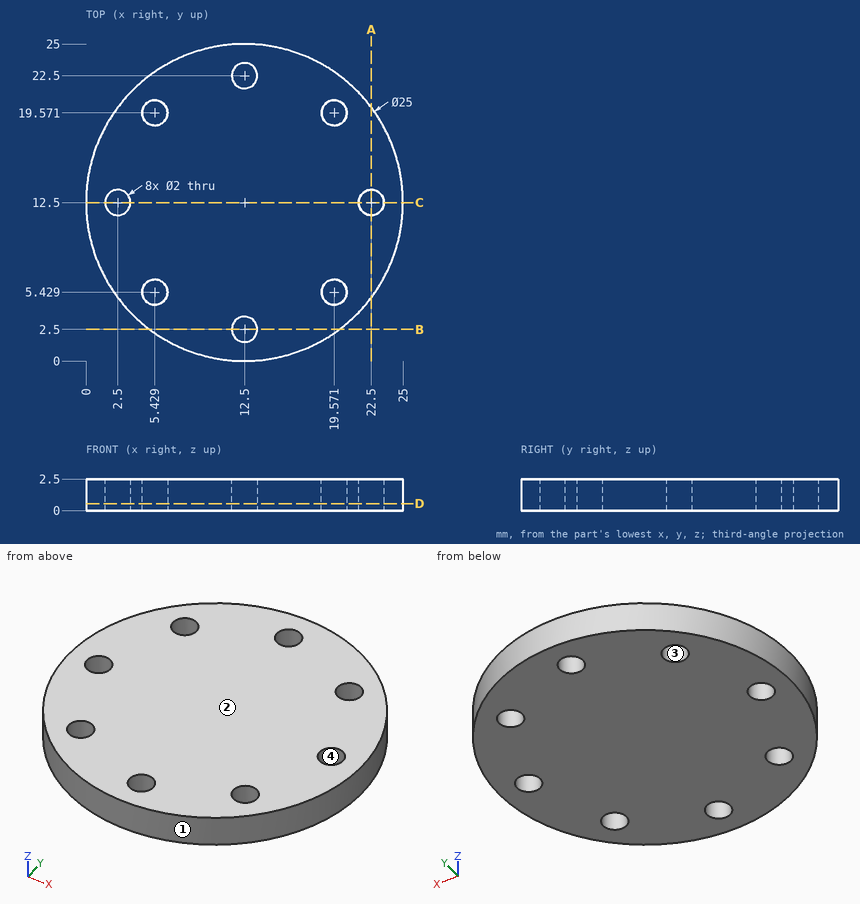
Geometry check sheet. Reference: drawing and pictorial views, mm from the part's lowest x, y, z. Give positions to 0.01 mm unless a question says otherwise; leave off trailing zeros. Order: outer loops, then holes, each group sorted by start corner. A loop starts at its lowest first (then second) coordinate and runs counter-clockwise, first axis right, second up.
1. Section check D-D, the plane z = 0.55. Give the number of separate pieces and of enclosed holes in the cut face, and give its area (3 significant figures).
2. Release check for a two-part mould opening along X. For the marked faces 1, 2, 3 and 4 record: pulls with the +X half, pulls with the -X half, needs draft (parallel to the pull), parting line crosses it, or undercut.
3. Thickness scan on L1, parallel to Y at x = 12.5, z = 0.25; L2, parallel to Y at x = 11.75, z = 0.2; L3, parallel to X at y = 18.75, z = 1.65 (1 decimal). Record the ranges inside material, lowest first.
4. Section check A-A, the plane x = 22.5. Enter the section's corners in (y, z), and give its area (3 significant figures).
5. Gauge pin test, flat end, axial feed: pin 1 Ø1 at (y, z) = (9.5, 1.5) entering from +X. Record the tip position at first contact, or that the pin passes through.
6. Section check C-C, the plane y = 12.5. Enter the section's corners in (x, z).
Values follow:
1. separate pieces: 1
1. enclosed holes: 8
1. area: 466 mm2
2. face 1: parting line crosses it
2. face 2: needs draft
2. face 3: undercut
2. face 4: undercut
3. L1: y = 0 to 1.5, 3.5 to 21.5, 23.5 to 25
3. L2: y = 0.02 to 1.84, 3.16 to 21.84, 23.16 to 24.98
3. L3: x = 1.7 to 4.9, 6 to 19, 20.1 to 23.3
4. outline: (5, 0) - (11.5, 0) - (11.5, 2.5) - (5, 2.5) - close; (13.5, 0) - (20, 0) - (20, 2.5) - (13.5, 2.5) - close
4. area: 32.5 mm2
5. pin 1: stops at x = 24.75
6. outline: (0, 0) - (1.5, 0) - (1.5, 2.5) - (0, 2.5) - close; (3.5, 0) - (21.5, 0) - (21.5, 2.5) - (3.5, 2.5) - close; (23.5, 0) - (25, 0) - (25, 2.5) - (23.5, 2.5) - close
